from build123d import *

# Parameters (mm, degrees)
SKETCH1_R           = 4.826
SKETCH1_R_2         = 1.5621
SKETCH1_R_3         = 4.0386
SKETCH1_W           = 12.7
SKETCH1_H           = 6.35
SKETCH1_W_2         = 6.35
SKETCH1_H_2         = 12.7
BOSS_EXTRUDE1_DEPTH = 6.35
SKETCH2_R           = 1.1303
CUT_EXTRUDE1_DEPTH  = 12.7
CHAMFER1_SIZE       = 1.905


with BuildPart() as part:
    # Sketch1 → Boss-Extrude1 (new body)
    with BuildSketch(Plane(origin=(0, 0, 0), x_dir=(1, 0, 0), z_dir=(0, 1, 0))):
        with BuildLine():
            Line((24.384, 81.026), (9.322766338, -1.952345462))
            ThreePointArc((9.322766338, -1.952345462), (0, -9.525), (-9.322766338, -1.952345462))
            ThreePointArc((-9.322766338, -1.952345462), (-10.68238726, 4.182597127), (-12.184698283, 10.284166696))
            Line((-12.184698283, 10.284166696), (-33.655, 81.026))
            Line((-33.655, 81.026), (-33.655, 112.776))
            Line((-33.655, 112.776), (-30.48, 112.776))
            Line((-30.48, 112.776), (24.384, 112.776))
            Line((24.384, 112.776), (24.384, 103.251))
            Line((24.384, 103.251), (30.734, 103.251))
            Line((30.734, 103.251), (30.734, 90.8558))
            Line((30.734, 90.8558), (24.384, 90.8558))
            Line((24.384, 90.8558), (24.384, 81.026))
        make_face()
        Circle(SKETCH1_R, mode=Mode.SUBTRACT)
        with Locations((-28.415132449, 107.954943271)):
            Circle(SKETCH1_R_2, mode=Mode.SUBTRACT)
        with Locations((-28.394285298, 85.856962938)):
            Circle(SKETCH1_R_2, mode=Mode.SUBTRACT)
        with Locations((-15.748, 100.8634)):
            Circle(SKETCH1_R_3, mode=Mode.SUBTRACT)
        with Locations((19.043196245, 96.393)):
            Circle(SKETCH1_R_2, mode=Mode.SUBTRACT)
        with BuildLine():
            Line((-5.032922832, 10.284166696), (-24.24305587, 73.5790401))
            ThreePointArc((-24.24305587, 73.5790401), (-23.396628753, 75.163136415), (-21.812532438, 74.316709298))
            Line((-21.812532438, 74.316709298), (-2.6023994, 11.021835893))
            ThreePointArc((-2.6023994, 11.021835893), (-3.448826517, 9.437739578), (-5.032922832, 10.284166696))
        make_face(mode=Mode.SUBTRACT)
        with Locations((7.994206079, 96.393)):
            Rectangle(SKETCH1_W, SKETCH1_H, mode=Mode.SUBTRACT)
        with Locations((-28.415132449, 96.901)):
            Rectangle(SKETCH1_W_2, SKETCH1_H_2, mode=Mode.SUBTRACT)
    extrude(amount=BOSS_EXTRUDE1_DEPTH)

    # Sketch2 → Cut-Extrude1 (cut)
    with BuildSketch(Plane(origin=(24.384, 0, 0), x_dir=(0, 0, -1), z_dir=(1, 0, 0))):
        with Locations((108.0135, 3.175)):
            Circle(SKETCH2_R)
        with Locations((85.9155, 3.175)):
            Circle(SKETCH2_R)
    extrude(amount=-CUT_EXTRUDE1_DEPTH, mode=Mode.SUBTRACT)

    # Chamfer1
    chamfer1_edges = [part.edges().sort_by_distance(p)[0] for p in [
        (17.481096245, 6.35, -96.393),
        (-29.977232449, 6.35, -107.954943271),
        (-29.956385298, 6.35, -85.856962938),
    ]]
    chamfer(chamfer1_edges, length=CHAMFER1_SIZE)


solid = part.part
Source: CAD feature listing. Evaluate the final solid. Frame: model axes, mm. A direction names the side the tool comes from. Coordinates: 2 decimals unless noted, no trailing zeros. Loops run counter-clockwise (first coordinate to the right, second up) from the corner with the lowest first, then second, coordinate; pieces in that order, holes last. Notation, with made-up numbers: (80, 33.5) - (85, 33.5) arc R20 cw to (85, 62.5) - close; hole circle Ø1 at (-8, -39). An arc over 180 degrees is marked (long way). Return JSON: item names as keys, results as strings.
Q1. Mould query, pull axis X, two halves, no side actions, for faces 1 (the flat face through (30.734, 3, -97)), 2 (the cylindrical face through (18.84, 2.19, -97.94)), 3 (the cylindrical face through (-10.662, 3.131, -4.097)). Classes: released by +X, released by -X, zero draft, split by the parting line, or undercut.
Results:
{"face 1": "released by +X", "face 2": "undercut", "face 3": "released by -X"}
Q2. Material intervals for line 1 along X through (y, z) = (1, -94) (3 decimals); line 2 along X through (y, z) = (3.5, -91) (3 decimals); line 3 along X through (y, z) = (1.25, -95.5) (3 decimals), sorted ascending.
Results:
{"line 1": "-33.655 to -31.59, -25.24 to 1.644, 14.344 to 30.734", "line 2": "-33.655 to -31.59, -25.24 to 30.734", "line 3": "-33.655 to -31.59, -25.24 to 1.644, 14.344 to 17.762, 20.325 to 30.734"}
Q3. Access query for faces 4 (the flat face through (-25.24, 3, -97)), 5 (the flat face through (24.384, 4, -87)), 6 (the flat face through (-22.77, 3.13, -45.16)), 7 (the cylindrical face through (18.123, 3.515, -109.092)). Directions: +Z, -Z, +X, -X, +Y, -Y. A direction counts if a zero-diameter tool reaches every point of the face in a straight line with its end or side. Return the directions, or none.
Results:
{"face 4": "+Y, -Y", "face 5": "+Z, +X, +Y, -Y", "face 6": "+Z, -X, +Y, -Y", "face 7": "+X"}
Q4. Contact query for flat-ended pins moving along their axis: P1, Ø1, axis at y = 1, z = -26.5, coming from the -X side; P2, Ø1.8, axis at y = 3, z = -86.5, coming from the +X side; P3, Ø4, axis at x = -28.42, z = -107.95, coming from the +Y side. Output: stop coordinate, or through.
Results:
{"P1": "x = -17.26", "P2": "x = 24.38", "P3": "y = 4.89"}
Q5. Section C-C, the plane x = -17. Return loops of the section in (y, z).
Results:
{"outline": "(0, -112.78) - (6.35, -112.78) - (6.35, -104.7) - (0, -104.7) - close; (0, -97.02) - (6.35, -97.02) - (6.35, -58.46) - (0, -58.46) - close; (0, -49.71) - (6.35, -49.71) - (6.35, -26.15) - (0, -26.15) - close"}
Q6. Section B-B, the plane z = 0. Return loops of the section in (x, y).
Results:
{"outline": "(-9.74, 0) - (-4.83, 0) - (-4.83, 6.35) - (-9.74, 6.35) - close; (4.83, 0) - (9.68, 0) - (9.68, 6.35) - (4.83, 6.35) - close"}
Q7. Section A-A, the plane x = 0. Return loops of the section in (y, z) (3 decimals), plus the area to 3 significant figures.
Results:
{"outline": "(0, -112.776) - (6.35, -112.776) - (6.35, -4.826) - (0, -4.826) - close; (0, 4.826) - (6.35, 4.826) - (6.35, 9.525) - (0, 9.525) - close", "area": "715 mm2"}
